Here's how the part is built. I have some questions about the finished solid (model axes, mm). A direction names the side the tool comes from. Coordinates: 2 decimals unless noted, no trailing zeros. Order: outer loops, then holes, each group sorted by start corner. A loop starts at its lowest first (then second) coordinate and runs counter-clockwise, first axis right, second up. Notation, with made-up numbers: (40, -16.5) -> (54, -16.5) arc R18 cw to (54, 4.5) -> close; hole circle Ø2 at (-39.5, 71). An arc over 180 degrees is marked (long way). One line per item, written item: value. Start each with the question number.
```python
from build123d import *

# Parameters (mm, degrees)
F1_DEPTH = 60
F2_DEPTH = 30
F0_W     = 30
F0_H     = 60
F3_DEPTH = 10


with BuildPart() as f1:
    # F0 (on Front) → F1 (new body)
    with BuildSketch(Plane.XZ):
        Polygon((42.81108, -30.305127), (42.81108, 29.694873), (3.14041, 29.694873), (3.14041, -10.305127), (-17.079143, -10.305127), (-17.18892, -30.305127), (-7.18892, -30.305127), (-7.18892, -20.305127), (32.81108, -20.305127), (32.81108, -30.305127), align=None)
    extrude(amount=F1_DEPTH)

    # F0 (on Front) → F2 (join)
    with BuildSketch(Plane.XZ):
        Polygon((3.14041, -10.305127), (3.14041, 29.694873), (-16.85959, 29.694873), (-17.079143, -10.305127), align=None)
    extrude(amount=F2_DEPTH)

    # F0 (on Front) → F3 (join)
    with BuildSketch(Plane.XZ):
        with Locations((57.81108, -0.305127)):
            Rectangle(F0_W, F0_H)
    extrude(amount=F3_DEPTH)


solid = f1.part
```
Q1. If we mould it in two halves opening along X, with no side actions, what happens to faces 5 (the face through (-7, -30, 10)), 6 (the face through (42.811, -35, -1)), 7 (the face through (3.14, -45, 10)), 8 (the face through (-7.189, -30, -25))? For each: +X half, -X half, draft (parallel to the pull), parting line (faces both ways), or undercut.
Q2. Imagine slicing it at D-D (y = -15). Write out the boundary of the cut face in (x, z), plus the area to 3 significant figures.
Q3. Imagine slicing it at B-B (z = -24). Write out the boundary of the cut face in (x, y).
Q4. Imagine slicing it at A-A (y = -44). Write out the boundary of the cut face in (x, z), plus the area to 3 significant figures.
Q5. For P1, Ø5, axis at x = -2, y = -46, coming from the +Z side; P2, Ø8, axis at y = -21, z = -21, coming from the +X side; P3, Ø10, axis at x = -10.5, z = 5.5, coming from the -Y side, each with a flat end and sliding along its axis, tell me the tip position at first contact or that it passes through.
Q6. Imagine slicing it at C-C (x = -6). Write out the boundary of the cut face in (y, z), plus the area to 3 significant figures.
Q7. For faces 1 (the face through (27, 0, 0)), 2 (the face through (32.811, -30, -25)), 3 (the face through (-7, -45, -10.305)), 4 (the face through (58, -10, 0)), which set-ups out of +Z, -Z, +X, -X, +Y, -Y let a thin tool reach every point of the face, with its end or its side?
Q8. I need wall thicknesses on line 1 (X direction, y = -32, z = -27.5); line 2 (X direction, y = -17.5, z = -11.5); line 3 (X direction, y = -48, z = 9). Which ranges of each line are inside material? Lowest first, please.
Completed:
1. face 5: draft
1. face 6: +X half
1. face 7: -X half
1. face 8: undercut
2. outline: (-17.19, -30.31) -> (-7.19, -30.31) -> (-7.19, -20.31) -> (32.81, -20.31) -> (32.81, -30.31) -> (42.81, -30.31) -> (42.81, 29.69) -> (-16.86, 29.69) -> close
2. area: 3,190 mm2
3. outline: (-17.15, -60) -> (-7.19, -60) -> (-7.19, 0) -> (-17.15, 0) -> close; (32.81, -60) -> (42.81, -60) -> (42.81, -10) -> (72.81, -10) -> (72.81, 0) -> (32.81, 0) -> close
4. outline: (-17.19, -30.31) -> (-7.19, -30.31) -> (-7.19, -20.31) -> (32.81, -20.31) -> (32.81, -30.31) -> (42.81, -30.31) -> (42.81, 29.69) -> (3.14, 29.69) -> (3.14, -10.31) -> (-17.08, -10.31) -> close
4. area: 2,390 mm2
5. P1: stops at z = -10.31
5. P2: stops at x = 42.81
5. P3: stops at y = -30
6. outline: (-60, -20.31) -> (0, -20.31) -> (0, 29.69) -> (-30, 29.69) -> (-30, -10.31) -> (-60, -10.31) -> close
6. area: 1,800 mm2
7. face 1: +Z, -Z, +X, -X, +Y
7. face 2: -Z, +Y, -Y
7. face 3: +Z, -X, -Y
7. face 4: +Z, -Z, +X, -Y
8. line 1: x = -17.17 to -7.19, 32.81 to 42.81
8. line 2: x = -17.09 to 42.81
8. line 3: x = 3.14 to 42.81
